Could you check a few things on this model? Use its own coordinates, in mm. A direction names the side the tool comes from. Coordinates: 2 decimals unless noted, no trailing zeros. Write each loop counter-clockwise with the first axis right and the second up, starting at its lowest first coordinate (ties: lowest second). Pieces come first, ordered by that corner, then holes. Notation, with made-up numbers: (67, -28) - (121, -28) arc R38 cw to (121, 10) - close; hole circle Ø5 at (2, -38.75). An arc over 180 degrees is marked (long way). Answer as a JSON object with one key per item and string values. Group by question number.
1) Will these pins go through, and if not, where does the flat tip stop? pin 1 Ø10 at (x, z) = (-5, -8) entering from -Y; pin 2 Ø1.3 at (x, z) = (-6.5, -7) entering from +Y; pin 3 Ø1 at (x, y) = (-3, 5.5) entering from -Z; pin 4 Ø0.8 at (x, y) = (7.5, 2) entering from -Z.
2) If we section it at D-D (y = 10.75): Write out the boundary of the cut face in (x, z).
3) We'd pull the mould along Z, two halves only. Please class faces 4 (the flat face through (7, 2, -8.2)), 5 (the cylindrical face through (7.26, 2.963, -10.172)), 6 (the flat face through (1, 0.5, -2)): released by +Z, released by -Z, zero draft, split by the parting line, or undercut.
4) If we section it at B-B (z = -11): Write out the boundary of the cut face in (x, y), plus the area to 3 significant figures.
5) If we section it at A-A (y = 7): Write out the boundary of the cut face in (x, z).
6) Please list where these lines run through material, in increasing order: line 1 along X through (y, z) = (2.25, -9.75); line 2 along X through (y, z) = (3, -6.95); line 3 along Y through (x, z) = (7.5, -10.9).
7) On a 3-axis mill with a long thin cutter (end or side, diameter ignored), from which of +Z, -Z, +X, -X, +Y, -Y can I reach the whole of each face in a straight line? I mean faces 1 (the flat face through (0, 4.25, -11)), 2 (the cylindrical face through (-0.54, 1.26, 2.44)), 3 (the cylindrical face through (-9.626, 3.415, -11.346)). Say none if no direction works.
Autodesk Inventor part; units mm, degrees
ref_plane "YZ Plane" through (0, 0, 0) normal (1, 0, 0) x (0, 1, 0)
ref_plane "XZ Plane" through (0, 0, 0) normal (0, 1, 0) x (-1, 0, 0)
ref_plane "XY Plane" through (0, 0, 0) normal (0, 0, 1) x (1, 0, 0)
sketch "Sketch1" plane through (0, 0, 0) normal (0, 1, 0) x (-1, 0, 0)
  line L0 (-5, 4.5) -> (5, 4.5)
  line L1 (10, -0.5) -> (10, -12.2)
  line L2 (10, -12.2) -> (-10, -12.2)
  line L3 (-10, -12.2) -> (-10, -0.5)
  line L4 (0, 0) -> (0, -71.875) construction
  arc A0 (10, -0.5) -> (5, 4.5) centre (5, -0.5) ccw
  arc A1 (-5, 4.5) -> (-10, -0.5) centre (-5, -0.5) ccw
  point P0 (-10, 4.5)
  point P1 (10, 4.5)
  dimension "d0" = 20
  dimension "d1" = 12.2
  dimension "d2" = 4.5
  dimension "d28" = 5
extrude "Extrusion1" add sketch "Sketch1" along normal blind 2
sketch "Sketch2" plane through (0, 2, 0) normal (0, 1, 0) x (1, 0, 0)
  circle A0 centre (0, 0) radius 2.5
  dimension "d6" = 5
extrude "Extrusion2" cut sketch "Sketch2" against normal blind 1.5
hole "Hole1" at (0, 0.5, 0) direction (0, -1, 0) diameter 3.5 end through all
sketch "Sketch7" plane through (0, 2, 0) normal (0, 1, 0) x (1, 0, 0)
  line L0 (15, 10.7) -> (-18, 10.7) construction
  line L1 (3.5, 10.7) -> (-1.7, 10.7) construction
  circle A0 centre (0, 0) radius 2.5
  line L2 (-10, 12.2) -> (-10, 0.5)
  arc A1 (-10, 0.5) -> (-5, -4.5) centre (-5, 0.5) ccw
  line L3 (-5, -4.5) -> (5, -4.5)
  arc A2 (5, -4.5) -> (10, 0.5) centre (5, 0.5) ccw
  line L4 (10, 0.5) -> (10, 12.2)
  line L5 (10, 12.2) -> (-10, 12.2)
  line L6 (10, 12.2) -> (-10, 12.2)
  line L7 (-10, 12.2) -> (-10, 9.2)
  line L8 (-10, 9.2) -> (10, 9.2)
  line L9 (10, 9.2) -> (10, 12.2)
  dimension "d44" = 10.7
  dimension "d57" = 3
extrude "Extrusion5" add sketch "Sketch7" along normal blind 2.25 contours L5 L4 L8 L2
sketch "Sketch9" plane through (0, 4.25, 0) normal (0, 1, 0) x (1, 0, 0)
  line L0 (-10, 12.2) -> (-10, 9.2)
  line L1 (-10, 9.2) -> (10, 9.2)
  line L2 (10, 9.2) -> (10, 12.2)
  line L3 (10, 12.2) -> (-10, 12.2)
  line L4 (0, 0) -> (0, 12.2) construction
  line L5 (-10, 10.7) -> (10, 10.7) construction
  line L6 (10, 0.5) -> (10, 12.2)
  point P0 (-1.7, 10.7)
  point P1 (3.5, 10.7)
  dimension "d58" = 3.5
  dimension "d59" = 1.7
hole "Hole5" at (-1.7, 4.25, -10.7) at (3.5, 4.25, -10.7) direction (0, -1, 0) diameter 1.22 end through all
sketch "Sketch10" plane through (0, 0, 0) normal (0, -1, 0) x (1, 0, 0)
  circle A0 centre (-1.7, -10.7) radius 0.61
  circle A1 centre (3.5, -10.7) radius 0.61
  circle A2 centre (0, 0) radius 1.75
  line L0 (-10, -12.2) -> (-10, -0.5)
  line L1 (10, -12.2) -> (-10, -12.2)
  line L2 (10, -0.5) -> (10, -12.2)
  arc A3 (10, -0.5) -> (5, 4.5) centre (5, -0.5) ccw
  line L3 (-5, 4.5) -> (5, 4.5)
  arc A4 (-5, 4.5) -> (-10, -0.5) centre (-5, -0.5) ccw
  line L4 (10, -0.5) -> (10, -9.2)
  line L5 (10, -6.95) -> (-10, -6.95) construction
  line L6 (-10, -12.2) -> (-10, -0.5)
  line L7 (0, 0) -> (0, -12.2) construction
  arc A5 (10, -6.95) -> (5.5, -6.95) centre (7.75, -6.95) ccw
  arc A6 (-5.5, -6.95) -> (-10, -6.95) centre (-7.75, -6.95) ccw
  line L8 (-10, -9.2) -> (10, -9.2)
  line L9 (10, -9.2) -> (-10, -9.2)
  arc A7 (5.5, -9.2) -> (10, -9.2) centre (7.75, -9.2) ccw
  line L10 (10, -6.95) -> (10, -9.2)
  line L11 (5.5, -6.95) -> (5.5, -9.2)
  line L12 (-10, -9.2) -> (-10, -6.95)
  line L13 (-5.5, -6.95) -> (-5.5, -9.2)
  circle A8 centre (-7.75, -9.2) radius 2.25
  circle A9 centre (7.75, -9.2) radius 2.25
  dimension "d67" = 5.25
  dimension "d68" = 2.25
sketch "Sketch12" plane through (0, 0, 0) normal (0, -1, 0) x (1, 0, 0)
  circle A0 centre (-1.7, -10.7) radius 0.61
  circle A1 centre (3.5, -10.7) radius 0.61
  circle A2 centre (0, 0) radius 1.75
  line L0 (-10, -12.2) -> (-10, -0.5)
  line L1 (10, -12.2) -> (-10, -12.2)
  line L2 (10, -0.5) -> (10, -12.2)
  arc A3 (10, -0.5) -> (5, 4.5) centre (5, -0.5) ccw
  line L3 (-5, 4.5) -> (5, 4.5)
  arc A4 (-5, 4.5) -> (-10, -0.5) centre (-5, -0.5) ccw
  circle A5 centre (7, 7) radius 3
  line L4 (10, -0.5) -> (10, -12.2)
  line L5 (10, -0.5) -> (10, 7)
  arc A6 (10, -0.5) -> (5, 4.5) centre (5, -0.5) ccw
  line L6 (-5, 4.5) -> (5.6879, 9.6979)
  line L7 (-5, 4.5) -> (5, 4.5)
  dimension "d86" = 7
  dimension "d87" = 7
extrude "Extrusion6" add sketch "Sketch12" against normal up to surface (2 mm away) contours L6 A5 A3 L3 | A3 A5 L5 | A5 A3 | A5 A3
fillet "Fillet2" radius 10 1 edges at (-5, 1, 4.5)
sketch "Sketch13" plane through (0, 2, 0) normal (0, 1, 0) x (1, 0, 0)
  arc A0 (5.6879, -9.6979) -> (10, -7) centre (7, -7) ccw
  circle A1 centre (7, -7) radius 3
  point P0 (0, 0)
extrude "Extrusion7" add sketch "Sketch13" along normal blind 9.15
hole "Hole8" at (7, 11.15, 7) direction (0, -1, 0) diameter 1.5 depth 6.6
sketch "Sketch14" plane through (7, 11.15, 7) normal (0, 1, 0) x (1, 0, 0)
  circle A0 centre (0, 0) radius 0.75
  circle A1 centre (0, 0) radius 3
  circle A2 centre (0, 0) radius 1.25
  point P0 (-7, 7)
  dimension "d102" = 2.5
extrude "Extrusion8" add sketch "Sketch14" along normal blind 0.3 contours A2
extrude "Extrusion9" add sketch "Sketch10" against normal blind 9 contours A8 L8 | L0 A6 L13 A8 | L8 A8 | A9 L11 A5 L2 | A7 L8 | L8 A9
sketch "Sketch11" plane through (10, 0, -12.2) normal (0, 0, -1) x (-1, 0, 0)
  line L0 (10, 0) -> (10, 4.25) construction
  line L1 (0, 0) -> (20, 0)
  line L2 (20, 0) -> (20, 4.25)
  line L3 (0, 4.25) -> (20, 4.25)
  line L4 (0, 0) -> (0, 4.25)
  line L5 (0, 0) -> (0, 4.25)
  line L6 (0, 2.2) -> (20, 2.2) construction
  point P0 (2.5, 2.2)
  point P1 (17.5, 2.2)
  dimension "d77" = 2.2
  dimension "d78" = 15
hole "Hole7" at (7.5, 2.2, -12.2) at (-7.5, 2.2, -12.2) direction (0, 0, 1) diameter 1.6 depth 4
sketch "Sketch15" plane through (0, 9, 0) normal (0, 1, 0) x (1, 0, 0)
  arc A0 (5.5, 6.95) -> (10, 6.95) centre (7.75, 6.95) ccw
  arc A1 (-10, 6.95) -> (-5.5, 6.95) centre (-7.75, 6.95) ccw
  point P0 (0, 0)
hole "Hole9" at (7.75, 9, -6.95) at (-7.75, 9, -6.95) direction (0, -1, 0) diameter 2 depth 8
fillet "Fillet3" radius 2.1 2 edges at (-5.5, 3.125, -9.2) (5.5, 3.125, -9.2)
fillet "Fillet4" radius 2 9 edges at (8.5912, 0, 9.5432) (1.0936, 0, 7.4635) (-4.7027, 0, 4.7383) (-8.8594, 0, 2.6788) (-10, 0, -3.725) (-10, 0, -10.7) (10, 0, -10.7) (10, 4.25, -10.7) (-10, 4.25, -10.7)
equation "\"d48\" = encoder_mount_height"
equation "\"d67\" = dist_screw_mount_point_1"
equation "\"d77\" = fingertip_mounting_dist_from_edge"
equation "\"shaft_to_encoder_mount_points\" = 10.7"
equation "\"encoder_mount_point_1\" = 3.5"
equation "\"encoder_mount_point_2\" = 1.7"
equation "\"dist_screw_mount_point_1\" = 5.25"
equation "\"dist_screw_mount_point_2\" = 2.25"
equation "\"fingertip_mount_spacing\" = 15"
equation "\"encoder_mount_height\" = 2.25"
equation "\"fingertip_mounting_dist_from_edge\" = 2.2"
properties part number "phalanx_3_housing_R"
Here are the results:
{
 "1": {"pin 1": "stops at y = 0", "pin 2": "stops at y = 9", "pin 3": "passes through", "pin 4": "stops at z = -8.2"},
 "2": {"outline": "(5.69, 9.7) arc R3 ccw (long way) to (10, 7) arc R3 ccw to start; hole circle Ø1.5 at (7, 7)"},
 "3": {"face 4": "released by -Z", "face 5": "zero draft", "face 6": "undercut"},
 "4": {"outline": "(-10, 2) arc R2 ccw to (-8, 0) - (-2.23, 0) - (-2.23, 4.25) - (-6.4, 4.25) - (-6.4, 9) - (-9.1, 9) - (-9.1, 3.92) arc R2 ccw to (-10, 2.25) - close; (-1.17, 0) - (2.97, 0) - (2.97, 4.25) - (-1.17, 4.25) - close; (4.03, 0) - (8, 0) arc R2 ccw to (10, 2) - (10, 2.25) arc R2 ccw to (9.1, 3.92) - (9.1, 9) - (6.4, 9) - (6.4, 4.25) - (4.03, 4.25) - close; hole circle Ø1.6 at (-7.5, 2.2); hole circle Ø1.6 at (7.5, 2.2)", "area": "94.4 mm²"},
 "5": {"outline": "(-10, -9.2) arc R2.25 ccw to (-5.5, -9.2) - (-5.5, -6.95) arc R2.25 ccw to (-10, -6.95) - close; (5.5, -9.2) arc R2.25 ccw to (10, -9.2) - (10, -6.95) arc R2.25 ccw to (5.5, -6.95) - close; (5.69, 9.7) arc R3 ccw (long way) to (10, 7) arc R3 ccw to start; hole circle Ø2 at (-7.75, -6.95); hole circle Ø1.5 at (7, 7); hole circle Ø2 at (7.75, -6.95)"},
 "6": {"line 1": "x = -10 to -8.3, -6.7 to 6.7, 8.3 to 10", "line 2": "x = -10 to -8.75, -6.75 to -5.5, 5.5 to 6.75, 8.75 to 10", "line 3": "y = 0 to 1.4, 3 to 9"},
 "7": {"face 1": "-Z, +Y", "face 2": "+Y", "face 3": "-Z, -X, +Y"}
}
